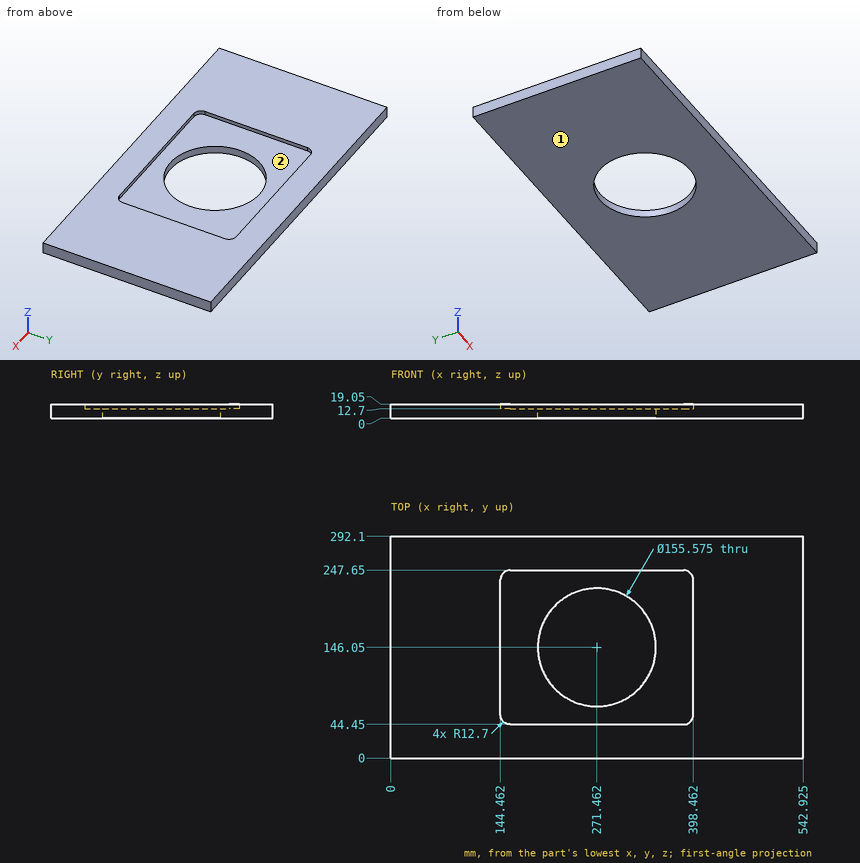
Can you work these out from the drawing? Everything is in mm from the part's minimum corner. Coordinates: 2 decimals unless noted, no trailing zeros.
1) Thinking about a two-plate mould opening in Y: for the marked faces 1 and 2, which applies, pulls with the +Y half, pulls with the -Y half, needs draft (parallel to the pull), parting line crosses it, or undercut?
2) For pin 1 (2 mm diameter, centred on x = 243, y = 53.5, fed in from +Z), with a flat end and sliding along its axis, tell me the tip position at first contact or that it passes through.
3) I need wall thicknesses on probe 1 along X at (y, z) = (197, 16.75) (1 decimal); probe 2 along Y at (x, z) = (257, 3.5); probe 3 along X at (y, z) = (135, 2.5) (1 decimal). Which ranges of each line are inside material? Lowest first, please.
Completed:
1. face 1: needs draft
1. face 2: undercut
2. pin 1: stops at z = 12.7
3. probe 1: x = 0 to 144.5, 398.5 to 542.9
3. probe 2: y = 0 to 69.62, 222.48 to 292.1
3. probe 3: x = 0 to 194.5, 348.5 to 542.9
